Geometry: final body of the model. Coordinates: model frame, mm. A direction names the side the tool comes from. Round coordinates to 2 decimals unless told otherwise and drop trailing zeros. Write each loop counter-clockwise with the first axis right and the second up, starting at its lowest first coordinate (ties: lowest second). Pieces come first, ordered by that corner, then holes. Notation, with made-up numbers: (-17, -10) -> (-8, -10) arc R15 ccw to (-8, 7) -> close; hole circle Ø6 at (71.5, 80). An arc over 180 degrees is marked (long way). Use one line per item in the form item = value. Start each with the question number.
1. Cut plane D-D, the plane z = 14.5. Return the cut outline in (x, y), plus the area to 3 significant figures.
2. Cut plane B-B, the plane x = 5.5. Return the cut outline in (y, z) (3 decimals).
3. Pin query (flat end, axial travel): pin 1 Ø2 at (y, z) = (20, 15.5) entering from +X. Return the tip coordinate at first contact, or that it passes through.
4. Cut plane C-C, the plane z = 28. Return the cut outline in (x, y).
5. Reachability of faces 1 (the face through (8.2, 23.1, 15)), 2 (the face through (6, 40, 9.125)), 3 (the face through (3, 18.6, 15)), 4 (the face through (2.5, 40, 4)) from +Z, -Z, +X, -X, +Y, -Y: full face, straight path, thin tool, end or side. Return the list, or none.
6. Line query: L1, parallel to Z at x = 8.75, y = 41.5 (3 decimals); L2, parallel to X at y = 39.5, z = 4; L3, parallel to Y at x = 6.25, z = 21. Output: solid intervals per line, ascending.
7. Draft query along Z for faces 5 (the face through (3, 31, 32.25)), 6 (the face through (-2, 40, 9.125)), 7 (the face through (-2, 42.6, 27)), 8 (the face through (3, 31, -2)). Return one class per face: pulls with the +Z half, pulls with the -Z half, needs draft (parallel to the pull), parting line crosses it, or undercut.
8. Cut plane A-A, the plane y = 41. Return the cut outline in (x, z) (3 decimals), plus the area to 3 significant figures.
```python
from build123d import *

# Parameters (mm, degrees)
CYLINDER020_R     = 4.5
CYLINDER020_DEPTH = 4
BOX014_W          = 11.125
BOX014_H          = 6
BOX014_DEPTH      = 4
BOX015_W          = 11.125
BOX015_H          = 6
BOX015_DEPTH      = 4
BOX021_W          = 11.125
BOX021_H          = 6
BOX021_DEPTH      = 7.75
BOX003_W          = 14.25
BOX003_H          = 19
BOX003_DEPTH      = 34.25
BOX022_W          = 11.125
BOX022_H          = 6
BOX022_DEPTH      = 7.75


with BuildPart() as cylinder020:
    # Cylinder020 → Cylinder020 (new body)
    with BuildSketch(Plane(origin=(6.25, 18.6, 15.125), x_dir=(0, 0, -1), z_dir=(1, 0, 0))):
        Circle(CYLINDER020_R)
    extrude(amount=CYLINDER020_DEPTH)


with BuildPart() as base_holder:
    # Box014 → Box014 (new body)
    with BuildSketch(Plane(origin=(0, 36.6, -2), x_dir=(0, 0, 1), z_dir=(-1, 0, 0))):
        with Locations((5.5625, 3)):
            Rectangle(BOX014_W, BOX014_H)
    extrude(amount=BOX014_DEPTH)


with BuildPart() as base_holder001:
    # Box015 → Box015 (new body)
    with BuildSketch(Plane(origin=(-4, 36.6, 32.25), x_dir=(0, 0, -1), z_dir=(1, 0, 0))):
        with Locations((5.5625, 3)):
            Rectangle(BOX015_W, BOX015_H)
    extrude(amount=BOX015_DEPTH)


with BuildPart() as base_holder002:
    # Box021 → Box021 (new body)
    with BuildSketch(Plane(origin=(2.5, 36.6, 32.25), x_dir=(0, 0, -1), z_dir=(1, 0, 0))):
        with Locations((5.5625, 3)):
            Rectangle(BOX021_W, BOX021_H)
    extrude(amount=BOX021_DEPTH)


with BuildPart() as f_3d_print_syringe_holder:
    # Box003 → Box003 (new body)
    with BuildSketch(Plane(origin=(-4, 18.6, -2), x_dir=(1, 0, 0), z_dir=(0, 0, 1))):
        with Locations((7.125, 9.5)):
            Rectangle(BOX003_W, BOX003_H)
    extrude(amount=BOX003_DEPTH)


with BuildPart() as cut007:
    # Box022 → Box022 (new body)
    with BuildSketch(Plane(origin=(2.5, 36.6, 9.125), x_dir=(0, 0, -1), z_dir=(1, 0, 0))):
        with Locations((5.5625, 3)):
            Rectangle(BOX022_W, BOX022_H)
    extrude(amount=BOX022_DEPTH)

    # Fusion010: union base_holder, base_holder001, base_holder002, 3D_print_syringe_holder
    add(base_holder.part)
    add(base_holder001.part)
    add(base_holder002.part)
    add(f_3d_print_syringe_holder.part)

    # Cut007: cut Cylinder020
    add(cylinder020.part, mode=Mode.SUBTRACT)


solid = cut007.part
```
Outcome:
q1.outline = (-4, 18.6) -> (6.25, 18.6) -> (6.25, 23.06) -> (10.25, 23.06) -> (10.25, 37.6) -> (-4, 37.6) -> close
q1.area = 253 mm^2
q2.outline = (18.6, -2) -> (42.6, -2) -> (42.6, 9.125) -> (37.6, 9.125) -> (37.6, 21.125) -> (42.6, 21.125) -> (42.6, 32.25) -> (18.6, 32.25) -> close
q3.pin_1 = 6.25
q4.outline = (-4, 18.6) -> (10.25, 18.6) -> (10.25, 42.6) -> (2.5, 42.6) -> (2.5, 37.6) -> (0, 37.6) -> (0, 42.6) -> (-4, 42.6) -> close
q5.face_1 = +X, -Y
q5.face_2 = +X, -X, +Y
q5.face_3 = +Z, -Z, +X, -X, -Y
q5.face_4 = +Z, -Z, +Y
q6.L1 = -2 to 9.125, 21.125 to 32.25
q6.L2 = -4 to 0, 2.5 to 10.25
q6.L3 = 18.6 to 37.6
q7.face_5 = pulls with the +Z half
q7.face_6 = undercut
q7.face_7 = needs draft
q7.face_8 = pulls with the -Z half
q8.outline = (-4, -2) -> (0, -2) -> (0, 9.125) -> (-4, 9.125) -> close; (-4, 21.125) -> (0, 21.125) -> (0, 32.25) -> (-4, 32.25) -> close; (2.5, -2) -> (10.25, -2) -> (10.25, 9.125) -> (2.5, 9.125) -> close; (2.5, 21.125) -> (10.25, 21.125) -> (10.25, 32.25) -> (2.5, 32.25) -> close
q8.area = 261 mm^2
